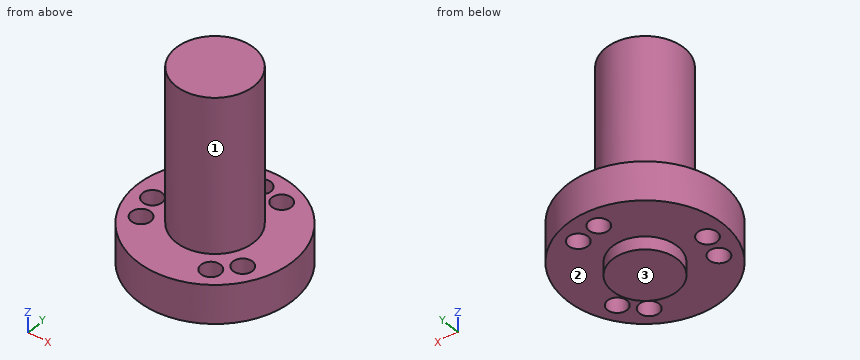
```python
from build123d import *

# Parameters (mm, degrees)
SKETCH_1_R      = 2.5
EXTRUDE_1_DEPTH = 1
SKETCH_2_R      = 6
SKETCH_2_R_2    = 0.75
EXTRUDE_2_DEPTH = 3
SKETCH_3_R      = 3
EXTRUDE_3_DEPTH = 12


with BuildPart() as part:
    # 草图1 → 凸台-拉伸1 (new body)
    with BuildSketch(Plane.XY):
        Circle(SKETCH_1_R)
    extrude(amount=EXTRUDE_1_DEPTH)

    # 草图2 → 凸台-拉伸2 (add)
    with BuildSketch(Plane.XY.offset(1)):
        Circle(SKETCH_2_R)
        with Locations((0, 4.5)):
            Circle(SKETCH_2_R_2, mode=Mode.SUBTRACT)
        with Locations((1.901782178, 4.078385042)):
            Circle(SKETCH_2_R_2, mode=Mode.SUBTRACT)
        with Locations((3.897114317, -2.25)):
            Circle(SKETCH_2_R_2, mode=Mode.SUBTRACT)
        with Locations((2.581093964, -3.686184199)):
            Circle(SKETCH_2_R_2, mode=Mode.SUBTRACT)
        with Locations((-3.897114317, -2.25)):
            Circle(SKETCH_2_R_2, mode=Mode.SUBTRACT)
        with Locations((-4.482876141, -0.392200842)):
            Circle(SKETCH_2_R_2, mode=Mode.SUBTRACT)
    extrude(amount=EXTRUDE_2_DEPTH)

    # 草图3 → 凸台-拉伸3 (add)
    with BuildSketch(Plane.XY.offset(4)):
        Circle(SKETCH_3_R)
    extrude(amount=EXTRUDE_3_DEPTH)


solid = part.part
```
Verification items for the finished model (mm, model axes). Face numbers are marked on the shaded views. A direction names the side the tool comes from. Give positions to 0.01 mm unless a question says otherwise; leave off trailing zeros. Order: outer loops, then holes, each group sorted by start corner. A loop starts at its lowest first (then second) coordinate and runs counter-clockwise, first axis right, second up. Notation, with made-up numbers: (-26, 49) -> (-7, 49) arc R27 cw to (-7, 69) -> close; hole circle Ø2 at (46, 81). An arc over 180 degrees is marked (long way). One line per item, written item: value.
(1) Gauge pin test, flat ends, axial feed: pin 1 (3 mm diameter, centred on x = -1, z = 2, fed in from +Y); pin 2 (2 mm diameter, centred on x = -3.5, z = 3.5, fed in from +Y); pin 3 (2 mm diameter, centred on x = 2.5, y = -4.5, fed in from -Z). Record the tip position at first contact, or that the pin passes through.
Final values:
pin 1: y = 6
pin 2: y = 5.45
pin 3: z = 1
(2) Sectioned sample at B-B on z = 2.5. Record the cut outline in (x, y), then the cut area to 3 significant figures.
Final values:
outline: circle Ø12 at (0, 0); hole circle Ø1.5 at (-4.48, -0.39); hole circle Ø1.5 at (-3.9, -2.25); hole circle Ø1.5 at (0, 4.5); hole circle Ø1.5 at (1.9, 4.08); hole circle Ø1.5 at (2.58, -3.69); hole circle Ø1.5 at (3.9, -2.25)
area: 102 mm^2
(3) Scan lines: line 1 along Y through (x, z) = (0, 3.45); line 2 along Z through (x, y) = (-2.5, 4.5); line 3 along X through (y, z) = (-4.25, 3.5). Record each from-to range of solid material in increasing order. Write a range as [from, to].
Final values:
line 1: [-6, 3.75], [5.25, 6]
line 2: [1, 4]
line 3: [-4.24, 2.09], [3.08, 4.24]
(4) Sectioned sample at C-C on y = 0. Record the cut outline in (x, z), then the cut area to 3 significant figures.
Final values:
outline: (-6, 1) -> (-5.12, 1) -> (-5.12, 4) -> (-6, 4) -> close; (-3.84, 1) -> (-2.5, 1) -> (-2.5, 0) -> (2.5, 0) -> (2.5, 1) -> (6, 1) -> (6, 4) -> (3, 4) -> (3, 16) -> (-3, 16) -> (-3, 4) -> (-3.84, 4) -> close
area: 109 mm^2
(5) Sectioned sample at D-D on y = 4.5. Record the cut outline in (x, z), then the cut area to 3 significant figures.
Final values:
outline: (-3.97, 1) -> (-0.75, 1) -> (-0.75, 4) -> (-3.97, 4) -> close; (0.75, 1) -> (1.28, 1) -> (1.28, 4) -> (0.75, 4) -> close; (2.52, 1) -> (3.97, 1) -> (3.97, 4) -> (2.52, 4) -> close
area: 15.6 mm^2
(6) Sectioned sample at A-A on x = 0. Record the cut outline in (y, z), then the cut area to 4 significant figures.
Final values:
outline: (-6, 1) -> (-2.5, 1) -> (-2.5, 0) -> (2.5, 0) -> (2.5, 1) -> (3.75, 1) -> (3.75, 4) -> (3, 4) -> (3, 16) -> (-3, 16) -> (-3, 4) -> (-6, 4) -> close; (5.25, 1) -> (6, 1) -> (6, 4) -> (5.25, 4) -> close
area: 108.5 mm^2
(7) Tool access check on the marked faces 1, 2 and 3. Record the directions out of +Z, -Z, +X, -X, +Y, -Y that give a thin tool (end or side, any length) a straight path to the whole face; none if there is none.
Final values:
face 1: +Z
face 2: -Z
face 3: -Z, +X, -X, +Y, -Y
